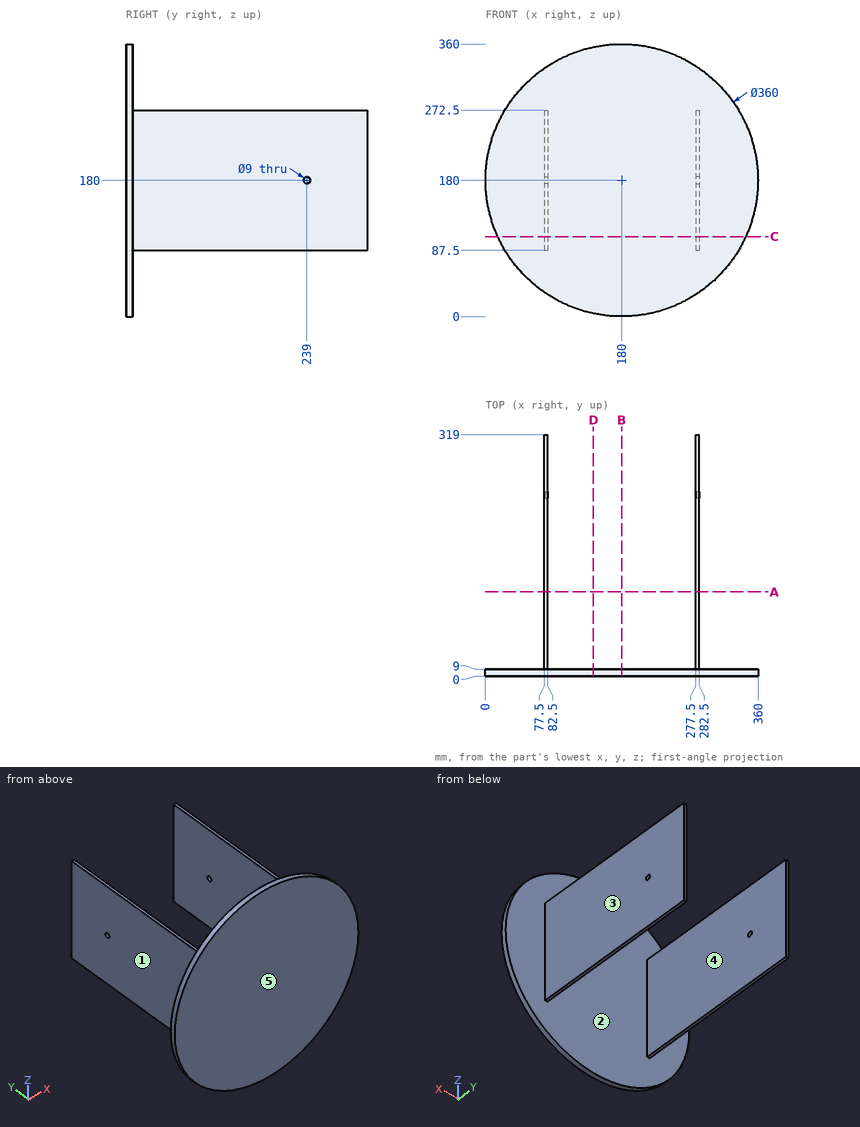
Input: dimensioned drawing with shaded views. Units: mm. Origin: part minimum x, y, z. A direction names the side the tool comes from. Round coordinates to 2 decimals unless told otherwise and drop trailing zeros. Loops run counter-clockwise (first coordinate to the right, second up) from the corner with the lowest first, then second, coordinate; pieces in that order, holes last. Notation, with made-up numbers: (-13.75, -10) -> (0.25, -10) arc R22 cw to (0.25, -2) -> close; hole circle Ø7 at (13, 73.25). An arc over 180 degrees is marked (long way). One line per item, written item: value.
(1) Section A-A (y = 111). Return the cut outline in (x, z), plus the area to 3 significant figures.
Geometry check:
outline: (77.5, 87.5) -> (82.5, 87.5) -> (82.5, 272.5) -> (77.5, 272.5) -> close; (277.5, 87.5) -> (282.5, 87.5) -> (282.5, 272.5) -> (277.5, 272.5) -> close
area: 1,850 mm2
(2) Mould query, pull axis X, two halves, no side actions, for the marked faces 1, 2 and 3. Classes: pulls with the +X half, pulls with the -X half, needs draft (parallel to the pull), parting line crosses it, or undercut.
Geometry check:
face 1: pulls with the -X half
face 2: undercut
face 3: pulls with the +X half
(3) Material intervals for line 1 (X direction, y = 305, z = 205); line 2 (Y direction, x = 279.95, z = 180); line 3 (Y direction, x = 259.5, z = 99), sorted ascending. Write a range as [from, to].
Geometry check:
line 1: [77.5, 82.5], [277.5, 282.5]
line 2: [0, 234.5], [243.5, 319]
line 3: [0, 9]
(4) Set-up query: the marked faces 4 and 5. Return all of +Z, -Z, +X, -X, +Y, -Y with unobstructed straight access to the full face (end or side cutting, diameter ignored); none if empty.
Geometry check:
face 4: +Z, -Z, +Y
face 5: +Z, -Z, +X, -X, -Y
(5) Section D-D (x = 142.5). Return the cut outline in (y, z).
Geometry check:
outline: (0, 3.95) -> (9, 3.95) -> (9, 356.05) -> (0, 356.05) -> close
(6) Section B-B (x = 180). Return the cut outline in (y, z), plus the area to 3 significant figures.
Geometry check:
outline: (0, 0) -> (9, 0) -> (9, 360) -> (0, 360) -> close
area: 3,240 mm2
(7) Section C-C (z = 105.5). Return the cut outline in (x, y).
Geometry check:
outline: (16.14, 0) -> (343.86, 0) -> (343.86, 9) -> (282.5, 9) -> (282.5, 319) -> (277.5, 319) -> (277.5, 9) -> (82.5, 9) -> (82.5, 319) -> (77.5, 319) -> (77.5, 9) -> (16.14, 9) -> close
(8) Pin query (flat end, axial travel): pin 1 (5.5 mm diameter, centred on x = 79.5, y = 96.5, fed in from +Z); pin 2 (5.5 mm diameter, centred on x = 280, y = 230.5, fed in from -Z); pin 3 (1.5 mm diameter, centred on x = 120, z = 220.5, fed in from +Y). Return the tip coordinate at first contact, or that it passes through.
Geometry check:
pin 1: z = 272.5
pin 2: z = 87.5
pin 3: y = 9
